Could you check a few things on this model? Use its own coordinates, in mm. Give positions to 0.01 mm unless a question says otherwise; leave off trailing zeros. Loops run counter-clockwise (first coordinate to the right, second up) from the corner with the lowest first, then second, coordinate; pieces in that order, holes last. Notation, with made-up numbers: M -39.75,-23 L -24.75,-23 A25 cw -24.75,12 Z; hole C 83.5,82.25 d6. An arc over 180 degrees is marked long. Return JSON: item names as keys, results as strings. Group by question number.
1. For pin 1 (2 mm diameter, centred on x = 10.5, z = 10, fed in from -Y); pin 2 (2 mm diameter, centred on y = 2, z = 15, fed in from -X); pin 3 (3.5 mm diameter, centred on x = -10.61, z = -10.61, fed in from -Y), each with a flat end and sliding along its axis, tell me the tip position at first contact or that it passes through.
2. If we section it at B-B (x = 0): Write out the boundary of the cut face in (y, z).
3. If we section it at C-C (y = 1.4): Write out the boundary of the cut face in (x, z).
4. Please list where these lines run through material, in increasing order: line 1 (Z direction, x = -1, y = 1.15); line 2 (Z direction, x = -1.5, y = 2.75); line 3 (X direction, y = 4.4, z = 14.5).
5. If we section it at A-A (z = 0): Write out the boundary of the cut face in (x, y), plus the area to 4 significant figures.
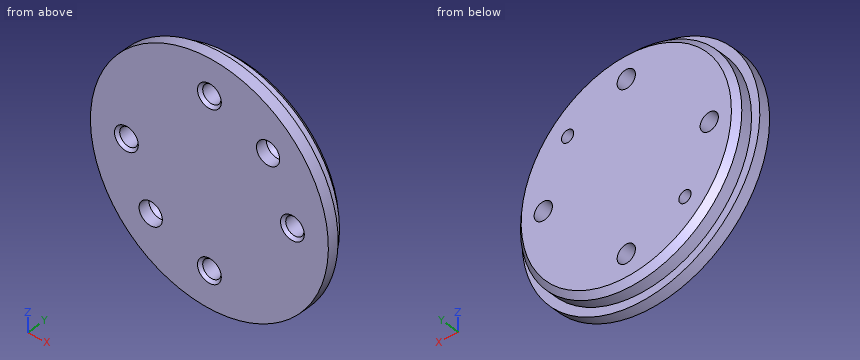
```python
from build123d import *

# Parameters (mm, degrees)
SKETCH_1_R                           = 21.5
EXTRUDE_1_DEPTH                      = 2
SKETCH_3_R                           = 20
EXTRUDE_2_DEPTH                      = 3
CHAMFER_1_SIZE                       = 1
SKETCH_4_R                           = 1.65
CUT_EXTRUDE_1_DEPTH                  = 31.813957876
CHAMFER_2_SIZE                       = 0.5
PATTERN_CIRCULAR_1_COUNT             = 4
CHAMFER_2_OF_PATTERN_CIRCULAR_1_SIZE = 0.5
SKETCH_5_R                           = 1.1
CUT_EXTRUDE_2_DEPTH                  = 31.813957876
SKETCH_6_R                           = 2.1
CUT_EXTRUDE_3_DEPTH                  = 2
CHAMFER_3_SIZE                       = 1
PATTERN_CIRCULAR_2_COUNT             = 2
CHAMFER_3_OF_PATTERN_CIRCULAR_2_SIZE = 1


with BuildPart() as part:
    # 草图1 → 凸台-拉伸1 (new body)
    with BuildSketch(Plane(origin=(0, 0, 0), x_dir=(1, 0, 0), z_dir=(0, 1, 0))):
        with Locations(Location((0, 0, 0), (0, 0, 270))):
            Circle(SKETCH_1_R)
    extrude(amount=EXTRUDE_1_DEPTH)

    # 草图3 → 凸台-拉伸2 (add)
    with BuildSketch(Plane(origin=(0, 2, 0), x_dir=(1, 0, 0), z_dir=(0, 1, 0))):
        with Locations(Location((0, 0, 0), (0, 0, 270))):
            Circle(SKETCH_3_R)
    extrude(amount=EXTRUDE_2_DEPTH)

    # 倒角1
    chamfer_1_edges = [part.edges().sort_by_distance(p)[0] for p in [
        (0, 5, -20),
    ]]
    chamfer(chamfer_1_edges, length=CHAMFER_1_SIZE)

    # 草图4 → 切除-拉伸1 (cut, through all)
    with BuildSketch(Plane(origin=(0, 5, 0), x_dir=(1, 0, 0), z_dir=(0, 1, 0))):
        with Locations(Location((0, 15, 0), (0, 0, 270))):
            Circle(SKETCH_4_R)
    cut_extrude_1 = extrude(amount=-CUT_EXTRUDE_1_DEPTH, mode=Mode.SUBTRACT)

    # 倒角2
    chamfer_2_edges = [part.edges().sort_by_distance(p)[0] for p in [
        (0, 0, -16.65),
    ]]
    chamfer(chamfer_2_edges, length=CHAMFER_2_SIZE)

    # 阵列(圆周)1: 切除-拉伸1 ×4 about axis
    pattern_circular_1_axis = Axis((0, 0, 0), (0, 1, 0))
    for i in range(1, PATTERN_CIRCULAR_1_COUNT):
        add(cut_extrude_1.rotate(pattern_circular_1_axis, i * 360 / PATTERN_CIRCULAR_1_COUNT), mode=Mode.SUBTRACT)

    # 倒角2 of 阵列(圆周)1
    chamfer_2_of_pattern_circular_1_edges = [part.edges().sort_by_distance(p)[0] for p in [
        (-16.65, 0, 0),
        (0, 0, 16.65),
        (16.65, 0, 0),
    ]]
    chamfer(chamfer_2_of_pattern_circular_1_edges, length=CHAMFER_2_OF_PATTERN_CIRCULAR_1_SIZE)

    # 草图5 → 切除-拉伸2 (cut, through all)
    with BuildSketch(Plane(origin=(0, 5, 0), x_dir=(1, 0, 0), z_dir=(0, 1, 0))):
        with Locations(Location((-10.606601718, 10.606601718, 0), (0, 0, 270))):
            Circle(SKETCH_5_R)
    cut_extrude_2 = extrude(amount=-CUT_EXTRUDE_2_DEPTH, mode=Mode.SUBTRACT)

    # 草图6 → 切除-拉伸3 (cut)
    with BuildSketch(Plane.XZ):
        with Locations(Location((-10.606601718, -10.606601718, 0), (0, 0, 270))):
            Circle(SKETCH_6_R)
    cut_extrude_3 = extrude(amount=-CUT_EXTRUDE_3_DEPTH, mode=Mode.SUBTRACT)

    # 倒角3
    chamfer_3_edges = [part.edges().sort_by_distance(p)[0] for p in [
        (-10.606601718, 2, -11.706601718),
    ]]
    chamfer(chamfer_3_edges, length=CHAMFER_3_SIZE - 0.0001)  # a hair under: the kernel refuses the full size

    # 阵列(圆周)2: 切除-拉伸2, 切除-拉伸3 ×2 about axis
    pattern_circular_2_axis = Axis((0, 0, 0), (0, 1, 0))
    add([cut_extrude_2.rotate(pattern_circular_2_axis, i * 360 / PATTERN_CIRCULAR_2_COUNT) for i in range(1, PATTERN_CIRCULAR_2_COUNT)], mode=Mode.SUBTRACT)
    add([cut_extrude_3.rotate(pattern_circular_2_axis, i * 360 / PATTERN_CIRCULAR_2_COUNT) for i in range(1, PATTERN_CIRCULAR_2_COUNT)], mode=Mode.SUBTRACT)

    # 倒角3 of 阵列(圆周)2
    chamfer_3_of_pattern_circular_2_edges = [part.edges().sort_by_distance(p)[0] for p in [
        (10.606601718, 2, 11.706601718),
    ]]
    chamfer(chamfer_3_of_pattern_circular_2_edges, length=CHAMFER_3_OF_PATTERN_CIRCULAR_2_SIZE - 0.0001)  # a hair under: the kernel refuses the full size


solid = part.part
```
Answer:
{
 "1": {"pin 1": "stops at y = 2.48", "pin 2": "stops at x = -16.32", "pin 3": "stops at y = 2.35"},
 "2": {"outline": "M 0,-21.5 L 2,-21.5 L 2,-20 L 4,-20 L 5,-19 L 5,-16.65 L 0.5,-16.65 L 0,-17.15 Z; M 0,-12.85 L 0.5,-13.35 L 5,-13.35 L 5,13.35 L 0.5,13.35 L 0,12.85 Z; M 0,17.15 L 0.5,16.65 L 5,16.65 L 5,19 L 4,20 L 2,20 L 2,21.5 L 0,21.5 Z"},
 "3": {"outline": "C 0,0 d43; hole C -15,0 d3.3; hole C -10.61,-10.61 d4.2; hole C 0,-15 d3.3; hole C 0,15 d3.3; hole C 10.61,10.61 d4.2; hole C 15,0 d3.3"},
 "4": {"line 1": "z = -21.48 to -16.31, -13.69 to 13.69, 16.31 to 21.48", "line 2": "z = -19.94 to -15.69, -14.31 to 14.31, 15.69 to 19.94", "line 3": "x = -13.19 to -1.57, 1.57 to 13.19"},
 "5": {"outline": "M -21.5,0 L -17.15,0 L -16.65,0.5 L -16.65,5 L -19,5 L -20,4 L -20,2 L -21.5,2 Z; M -13.35,0.5 L -12.85,0 L 12.85,0 L 13.35,0.5 L 13.35,5 L -13.35,5 Z; M 16.65,0.5 L 17.15,0 L 21.5,0 L 21.5,2 L 20,2 L 20,4 L 19,5 L 16.65,5 Z", "area": "171.5 mm²"}
}
